The figure shows three views and two pictorial views of one solid part (mm, origin at its lowest corner). Answer the questions. Coordinates: 2 decimals unless noted, no trailing zeros. Order: outer loops, then holes, each group sorted by start corner. A loop starts at its lowest first (then second) coordinate and runs counter-clockwise, first axis right, second up.
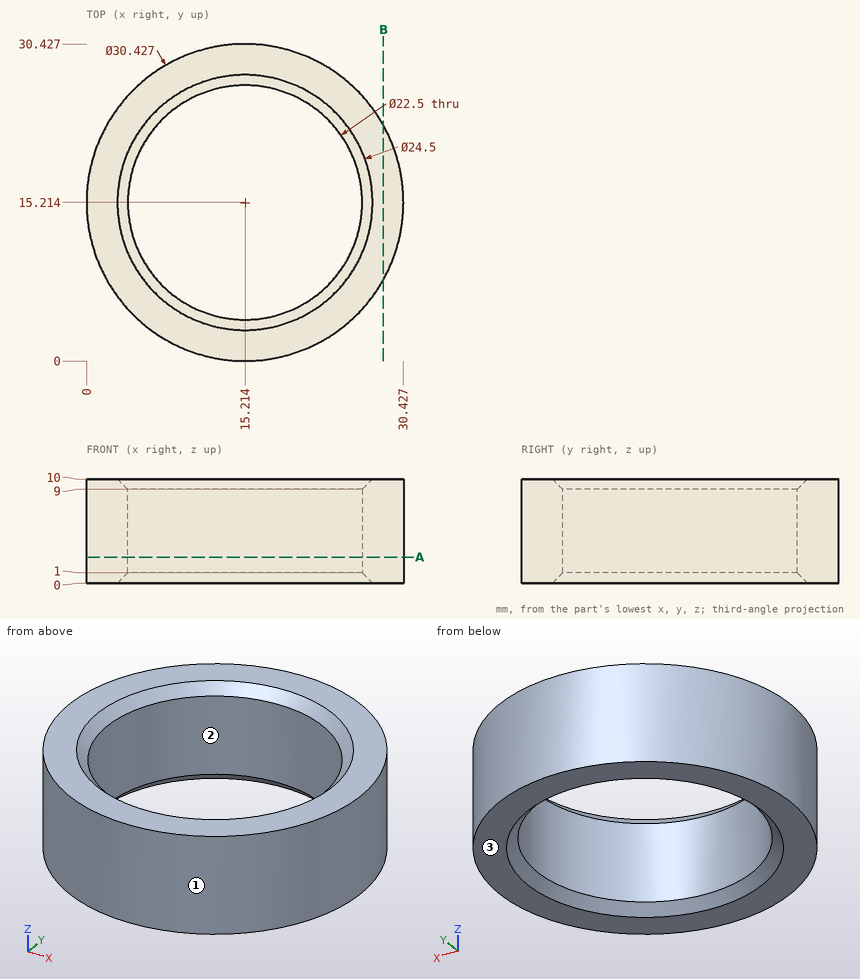
1) A cutting plane is placed at A-A, the plane z = 2.5. Write down the section's boundary in (x, y).
2) Straight lines are drawn through the part: probe 1 along Y at (x, z) = (12.5, 6.75) (1 decimal); probe 2 along X at (y, z) = (20, 4.75) (1 decimal); probe 3 along X at (y, z) = (24.5, 0.75) (1 decimal). For each, find the intervals that lie inside material, in ascending order.
3) The mould has two halves that part along Y. Classify the marked faces 1, 2 and 3: released by +Y, released by -Y, zero draft, split by the parting line, or undercut.
4) A cutting plane is placed at B-B, the plane x = 28.5. Write down the section's boundary in (y, z) (1 decimal).
5) Each of these flat-tipped pins is pushed along its axis until it touches: P1, Ø6, axis at x = 23, z = 3.5, coming from the -Y side; P2, Ø1.5, axis at y = 20.5, z = 8.5, coming from the +X side (1 decimal); P3, Ø8, axis at x = 7.5, y = 16, coming from the -Z side (1 decimal). Where does it stop, or does it pass through?
Working result:
1. outline: circle Ø30.43 at (15.21, 15.21); hole circle Ø22.5 at (15.21, 15.21)
2. probe 1: y = 0.2 to 4.3, 26.1 to 30.2
2. probe 2: x = 0.8 to 5, 25.4 to 29.7
2. probe 3: x = 3.2 to 8.4, 22 to 27.3
3. face 1: split by the parting line
3. face 2: undercut
3. face 3: zero draft
4. outline: (7.8, 0) - (22.6, 0) - (22.6, 10) - (7.8, 10) - close
5. P1: stops at y = 0.77
5. P2: stops at x = 29.7
5. P3: stops at z = 0.5
